from build123d import *

# Parameters (mm, degrees)
SKETCH1_R           = 11.1125
BOSS_EXTRUDE1_DEPTH = 7
BOSS_EXTRUDE2_DEPTH = 3
FILLET1_R           = 2


with BuildPart() as part:
    # Sketch1 → Boss-Extrude1 (new body)
    with BuildSketch(Plane(origin=(0, 0, 0), x_dir=(1, 0, 0), z_dir=(0, 1, 0))):
        Circle(SKETCH1_R)
        Polygon((6.35, 3.666174209), (0, 7.332348419), (-6.35, 3.666174209), (-6.35, -3.666174209), (0, -7.332348419), (6.35, -3.666174209), align=None, mode=Mode.SUBTRACT)
    extrude(amount=BOSS_EXTRUDE1_DEPTH)

    # Sketch2 → Boss-Extrude2 (add)
    with BuildSketch(Plane(origin=(0, 0, 0), x_dir=(1, 0, 0), z_dir=(0, 1, 0))):
        with BuildLine():
            Line((-4.7625, 111.640231571), (-12.7, 111.640231571))
            ThreePointArc((-12.7, 111.640231571), (-4.861835295, 121.90235174), (0, 133.865231571))
            ThreePointArc((0, 133.865231571), (4.861835295, 121.90235174), (12.7, 111.640231571))
            Line((12.7, 111.640231571), (4.7625, 111.640231571))
            Line((4.7625, 111.640231571), (4.7625, 10.040231571))
            Line((4.7625, 10.040231571), (-4.7625, 10.040231571))
            Line((-4.7625, 10.040231571), (-4.7625, 111.640231571))
        make_face()
    extrude(amount=BOSS_EXTRUDE2_DEPTH)

    # Fillet1
    fillet1_edges = [part.edges().sort_by_distance(p)[0] for p in [
        (0, 3, -11.1125),
        (-4.7625, 1.5, -111.640231571),
        (-4.7625, 1.5, -10.040231571),
        (4.7625, 1.5, -10.040231571),
        (4.7625, 1.5, -111.640231571),
        (12.7, 1.5, -111.640231571),
        (-12.7, 1.5, -111.640231571),
    ]]
    fillet(fillet1_edges, radius=FILLET1_R)


solid = part.part
For this review, take the finished solid that the model builds, in its own axes (mm). A direction names the side the tool comes from. Round coordinates to 2 decimals unless told otherwise and drop trailing zeros. Write each loop counter-clockwise with the first axis right and the second up, starting at its lowest first coordinate (ties: lowest second). Pieces come first, ordered by that corner, then holes. Notation, with made-up numbers: (-7, 76) -> (47, 76) arc R24 cw to (47, 94) -> close; hole circle Ø11 at (39.5, 60). An arc over 180 degrees is marked (long way). Use CSV: the item, a comma, the result in double quotes.
(1) Consider section A-A, the plane z = 0. Give the boundary of the cut face in (x, y).
Computed values:
outline,"(-11.11, 0) -> (-6.35, 0) -> (-6.35, 7) -> (-11.11, 7) -> close; (6.35, 0) -> (11.11, 0) -> (11.11, 7) -> (6.35, 7) -> close"
(2) Clearance check with flat-ended pins moving along their axes: P1, Ø6, axis at x = 5.5, z = -45.5, coming from the +Y side; P2, Ø4, axis at y = 3, z = -71, coming from the +X side; P3, Ø2, axis at y = 4.5, z = -1.5, coming from the -X side. State where each tip first meets the part, or that it passes through.
Computed values:
P1,"y = 3"
P2,"x = 4.76"
P3,"x = -11.1"
(3) For faces 4 (the face through (0, 3, -74)), 5 (the face through (-4.762, 2, -60)), 6 (the face through (3.219, 3.451, -5.474)), list the 3-axis set-ups (+Z, -Z, +X, -X, +Y, -Y) from which the entire face can be reached by the end or side of a thin tool; tool diameter is ignored.
Computed values:
face 4,"-Z, +X, -X, +Y"
face 5,"-X, +Y, -Y"
face 6,"+Y, -Y"
(4) Consider section B-B, the plane z = -106. Give the boundary of the cut face in (x, y), plus the area to 3 significant figures.
Computed values:
outline,"(-4.76, 0) -> (4.76, 0) -> (4.76, 3) -> (-4.76, 3) -> close"
area,"28.6 mm²"
(5) Draft analysis for pull direction X (two halves, no side actions). For faces 1 (the face through (-9.967, 1.521, -112.763)), 2 (the face through (4.762, 1, -61)), 3 (the face through (-6.35, 3, 0)), state which applies: +X half, -X half, draft (parallel to the pull), parting line (faces both ways), or undercut.
Computed values:
face 1,"-X half"
face 2,"+X half"
face 3,"undercut"
(6) To check wall thickness, follow L1, parallel to X at y = 1.5, z = -0.5; L2, parallel to Y at x = -1.75, z = -51.5; L3, parallel to Z at x = 7.25, y = 2.5. State the ranges of each line that lie inside material, in increasing order. Write a range as [from, to].
Computed values:
L1,"[-11.1, -6.35], [6.35, 11.1]"
L2,"[0, 3]"
L3,"[-118.14, -111.64], [-8.42, 8.42]"
